```python
from build123d import *

# Parameters (mm, degrees)
F1_DEPTH      = 10.16
F2_R          = 15.24
F3_DEPTH      = 7.62
F4_R          = 1.27
F5_R          = 8.89
F6_DEPTH      = 2.54
F6_DEPTH_BACK = 25.4
F7_R          = 5.6612408529
F8_DEPTH      = 15.241
F9_R          = 1.27
F11_DEPTH     = 15.24
F12_R         = 1.27
F13_R         = 12.573
F14_DEPTH     = 4.318
F15_R         = 5.8846996184
F16_DEPTH     = 21.083
F17_R         = 20.32
F18_DEPTH     = 10.80698
F20_DEPTH     = 25.4
F21_R         = 20.32
F3_FACE_R     = 13.97
F3_FACE_R_2   = 8.89
F22_DEPTH     = 10.8069888
F23_R         = 1.27


with BuildPart() as f1:
    # F0 (on Top) → F1 (new body)
    with BuildSketch(Plane.XY):
        with BuildLine():
            Line((0, 31.3225206132), (-39.7978979795, 67.4076240142))
            ThreePointArc((-39.7978979795, 67.4076240142), (-61.191545749, 67.9425235548), (-62.027639853, 46.5585288613))
            Line((-62.027639853, 46.5585288613), (-18.8440847739, -13.5402782767))
            ThreePointArc((-18.8440847739, -13.5402782767), (0, -23.2042812165), (18.8440847739, -13.5402782767))
            Line((18.8440847739, -13.5402782767), (62.027639853, 46.5585288613))
            ThreePointArc((62.027639853, 46.5585288613), (61.191545749, 67.9425235548), (39.7978979795, 67.4076240142))
            Line((39.7978979795, 67.4076240142), (0, 31.3225206132))
        make_face()
    extrude(amount=F1_DEPTH)

    # F2 (on face) → F3 (join)
    with BuildSketch(Plane.XY.offset(10.16)):
        with Locations((50.7659645325, 56.8265505295)):
            Circle(F2_R)
    extrude(amount=F3_DEPTH)

    # F4
    f4_edges = [f1.edges().sort_by_distance(p)[0] for p in [
        (35.525965, 56.826551, 17.78),
    ]]
    fillet(f4_edges, radius=F4_R)

    # F5 (on face) → F6 (cut, two sides)
    with BuildSketch(Plane.XY.offset(17.78)) as f6_sk:
        with Locations((50.7659645325, 56.8265505295)):
            Circle(F5_R)
    extrude(amount=-F6_DEPTH, mode=Mode.SUBTRACT)
    extrude(f6_sk.sketch, amount=F6_DEPTH_BACK, mode=Mode.SUBTRACT)

    # F7 (on face) → F8 (cut, through all)
    with BuildSketch(Plane.XY.offset(15.24)):
        with Locations((50.7659645325, 56.8265505295)):
            Circle(F7_R)
    extrude(amount=-F8_DEPTH, mode=Mode.SUBTRACT)

    # F9
    f9_edges = [f1.edges().sort_by_distance(p)[0] for p in [
        (0, 31.322521, 5.08),
    ]]
    fillet(f9_edges, radius=F9_R)

    # F10 (on face) → F11 (join)
    with BuildSketch(Plane.XY.offset(10.16)):
        with BuildLine():
            ThreePointArc((-62.027639853, 46.5585288613), (-45.260073682, 42.6158937557), (-35.5259645325, 56.8265505295))
            ThreePointArc((-35.5259645325, 56.8265505295), (-36.6342460548, 62.5319981777), (-39.7978979795, 67.4076240142))
            ThreePointArc((-39.7978979795, 67.4076240142), (-61.191545749, 67.9425235548), (-62.027639853, 46.5585288613))
        make_face()
    extrude(amount=F11_DEPTH)

    # F12
    f12_edges = [f1.edges().sort_by_distance(p)[0] for p in [
        (-61.734031, 46.245477, 25.4),
    ]]
    fillet(f12_edges, radius=F12_R)

    # F13 (on face) → F14 (cut)
    with BuildSketch(Plane.XY.offset(25.4)):
        with Locations((-50.7659645325, 56.8265505295)):
            Circle(F13_R)
    extrude(amount=-F14_DEPTH, mode=Mode.SUBTRACT)

    # F15 (on face) → F16 (cut, through all)
    with BuildSketch(Plane.XY.offset(21.082)):
        with Locations((-50.7659645325, 56.8265505295)):
            Circle(F15_R)
    extrude(amount=-F16_DEPTH, mode=Mode.SUBTRACT)

    # F17 (on face) → F18 (join)
    with BuildSketch(Plane.XY.offset(10.16)):
        Circle(F17_R)
    extrude(amount=F18_DEPTH)

    # F19 (on face) → F20 (cut)
    with BuildSketch(Plane.XY.offset(20.96698)):
        Polygon((5.08, 8.89), (-5.08, 8.89), (-9.9986888497, 0), (-5.08, -8.89), (5.08, -8.89), (9.9986888497, 0), align=None)
    extrude(amount=-F20_DEPTH, mode=Mode.SUBTRACT)

    # F21 (on face) + F3_face (on face) → F22 (join)
    with BuildSketch(Plane(origin=(0, 0, 0), x_dir=(1, 0, 0), z_dir=(0, 0, -1))):
        Circle(F21_R)
        Polygon((5.08, 8.89), (9.9986888497, 0), (5.08, -8.89), (-5.08, -8.89), (-9.9986888497, 0), (-5.08, 8.89), align=None, mode=Mode.SUBTRACT)
    with BuildSketch(Plane(origin=(50.7659645325, 56.8265505295, 17.78), x_dir=(1, 0, 0), z_dir=(0, 0, 1))):
        Circle(F3_FACE_R)
        Circle(F3_FACE_R_2, mode=Mode.SUBTRACT)
    extrude(amount=F22_DEPTH, dir=(0, 0, -1))

    # F23
    f23_edges = [f1.edges().sort_by_distance(p)[0] for p in [
        (-20.32, 0, 20.96698),
        (-20.32, 0, -10.806989),
    ]]
    fillet(f23_edges, radius=F23_R)


solid = f1.part
```
Geometry check sheet. Reference: the model listing, model coordinates, mm. A direction names the side the tool comes from. Coordinates: 2 decimals unless noted, no trailing zeros. Write each loop counter-clockwise with the first axis right and the second up, starting at its lowest first coordinate (ties: lowest second). Pieces come first, ordered by that corner, then holes. Notation, with made-up numbers: M 73.25,77.5 L 87.25,77.5 A18 ccw 87.25,107.5 Z; hole C -36,76.5 d1. An arc over 180 degrees is marked long. One line per item, written item: value. Start each with the question number.
(1) Depth check by flat-ended pin: pin 1 (18 mm diameter, centred on x = 50.77, y = 56.83, fed in from +Z); pin 2 (3 mm diameter, centred on y = 49.5, z = 8.5, fed in from -X); pin 3 (5 mm diameter, centred on y = 32, z = 9, fed in from +X). Enter the tip coordinate at first touch or a pass-through.
(2) Tool access check on faces 1 (the face through (-7.574, -4.383, 5.302)), 2 (the face through (-40.74, 16.93, 5.01)), 3 (the face through (-20.05, 49.5, 5.01)), 4 (the face through (57, 57, 15.24)). Record the directions out of +Z, -Z, +X, -X, +Y, -Y that give a thin tool (end or side, any length) a straight path to the whole face; none if there is none.
(3) Scan lines: line 1 along Z through (x, y) = (-26, 24.5); line 2 along X through (y, z) = (8.5, 14); line 3 along Y through (x, z) = (-7, 19). Record each from-to range of solid material in increasing order. Write a range as [from, to].
(4) Sectioned sample at A-A, the plane z = -2. Enter the section's corners in (x, y), and give its area (3 significant figures).
(5) Sectioned sample at B-B, the plane y = 39. Enter the section's corners in (x, z), and give its area (3 significant figures).
(6) Sectioned sample at C-C, the plane x = 29. Enter the section's corners in (y, z).
(7) Release check for a two-part mould opening along Y. For faces 5 (the face through (7.574, 4.383, 5.302)), 6 (the face through (20.6, 50, 5)), 7 (the face through (64.908, 62.507, 9.974)) record: released by +Y, released by -Y, zero draft, split by the parting line, or undercut.
Filled sheet:
1. pin 1: z = 17.78
1. pin 2: x = -64.85
1. pin 3: x = 53.36
2. face 1: +Z, -Z
2. face 2: +Z, -Z, -X, -Y
2. face 3: +Z, -Z, +Y
2. face 4: +Z
3. line 1: [0, 10.16]
3. line 2: [-18.46, -5.3], [5.3, 18.46]
3. line 3: [-19.08, -5.42], [5.42, 19.08]
4. outline: C 0,0 d40.64; hole M -10,0 L -5.08,-8.89 L 5.08,-8.89 L 10,0 L 5.08,8.89 L -5.08,8.89 Z
4. area: 1,030 mm²
5. outline: M -56.6,0 L -8.47,0 L -8.47,10.16 L -56.6,10.16 Z; M 8.47,0 L 56.6,0 L 56.6,10.16 L 8.47,10.16 Z
5. area: 978 mm²
6. outline: M 0.59,0 L 57.62,0 L 57.62,10.16 L 0.59,10.16 Z
7. face 5: undercut
7. face 6: released by +Y
7. face 7: split by the parting line
